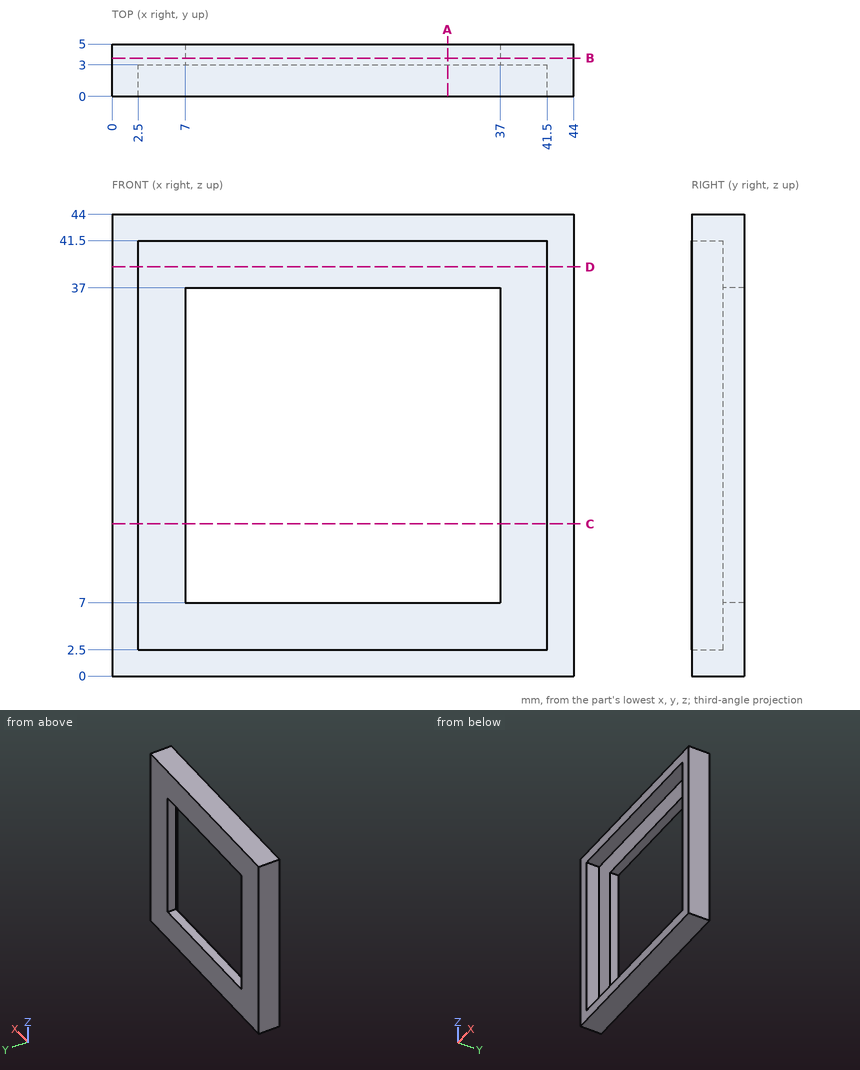
Here's the drawing with two shaded views (mm, measured from the low corner). I have some questions. Round coordinates to 2 decimals unless told otherwise and drop trailing zeros. Write each loop counter-clockwise with the first axis right and the second up, starting at its lowest first coordinate (ties: lowest second). Pieces come first, ordered by that corner, then holes. Notation, with made-up numbers: M -18.75,37.5 L 27.25,37.5 A8 ccw 27.25,42.5 Z; hole C 44,35.5 d1. An arc over 180 degrees is marked long. Use CSV: the item, a comma, the result in double quotes.
(1) Imagine slicing it at C-C (z = 14.5). Write out the boundary of the cut face in (x, y).
Check values:
outline,"M 0,0 L 2.5,0 L 2.5,3 L 7,3 L 7,5 L 0,5 Z; M 37,3 L 41.5,3 L 41.5,0 L 44,0 L 44,5 L 37,5 Z"
(2) I need wall thicknesses on line 1 along Z through (x, y) = (27.5, 3.95); line 2 along Z through (x, y) = (30.5, 2.25). Which ranges of each line are inside material? Lowest first, please.
Check values:
line 1,"0 to 7, 37 to 44"
line 2,"0 to 2.5, 41.5 to 44"
(3) I'm going to push a flat-ended pin straight in: pin 1 (1.5 mm diameter, centred on x = 19.5, z = 6, fed in from -Y). Where does the tip first touch, or does it pass through?
Check values:
pin 1,"y = 3"
(4) Imagine slicing it at B-B (y = 3.65). Write out the boundary of the cut face in (x, z), plus the area to 3 significant figures.
Check values:
outline,"M 0,0 L 44,0 L 44,44 L 0,44 Z; hole M 7,7 L 37,7 L 37,37 L 7,37 Z"
area,"1,040 mm^2"
(5) Imagine slicing it at A-A (x = 32). Write out the boundary of the cut face in (y, z), plus the area to 3 significant figures.
Check values:
outline,"M 0,0 L 5,0 L 5,7 L 3,7 L 3,2.5 L 0,2.5 Z; M 0,41.5 L 3,41.5 L 3,37 L 5,37 L 5,44 L 0,44 Z"
area,"43.0 mm^2"
(6) Imagine slicing it at D-D (z = 39). Write out the boundary of the cut face in (x, y), plus the area to 3 significant figures.
Check values:
outline,"M 0,0 L 2.5,0 L 2.5,3 L 41.5,3 L 41.5,0 L 44,0 L 44,5 L 0,5 Z"
area,"103 mm^2"
